from build123d import *

# Parameters (mm, degrees)
BOSS_EXTRUDE1_DEPTH = 3
BOSS_EXTRUDE2_DEPTH = 3
BOSS_EXTRUDE3_DEPTH = 3
BOSS_EXTRUDE4_DEPTH = 3


with BuildPart() as part:
    # Sketch1 → Boss-Extrude1 (new body)
    with BuildSketch(Plane.XY):
        Polygon((0, 0), (5, 1), (1.8, 5.5), (1.8, 1.5), (0, 1.5), align=None)
    extrude(amount=BOSS_EXTRUDE1_DEPTH)

    # Sketch2 → Boss-Extrude2 (add)
    with BuildSketch(Plane(origin=(0, 0, 0), x_dir=(-1, 0, 0), z_dir=(0, 0, -1))):
        Polygon((-5, 1), (-3.2, 3.53125), (-3.2, 1.5), (0, 1.5), (0, 0), align=None)
    extrude(amount=BOSS_EXTRUDE2_DEPTH)

    # Sketch3 → Boss-Extrude3 (add)
    with BuildSketch(Plane(origin=(0, 0, -3), x_dir=(-1, 0, 0), z_dir=(0, 0, -1))):
        Polygon((-3.2, 3.53125), (0, 1.5), (-3.2, 1.5), align=None)
    extrude(amount=-BOSS_EXTRUDE3_DEPTH)

    # Sketch4 → Boss-Extrude4 (add)
    with BuildSketch(Plane.XY):
        Polygon((1.8, 2.642578125), (1.8, 1.5), (0, 1.5), align=None)
    extrude(amount=BOSS_EXTRUDE4_DEPTH)


solid = part.part
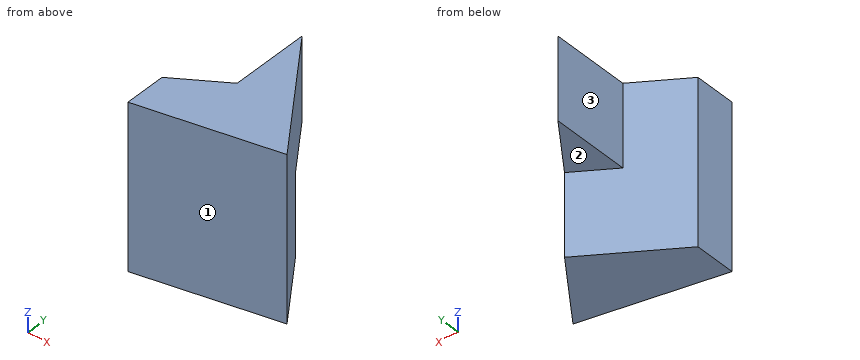
Part model, mm, in its own coordinate system. Face numbers are marked on the shaded views. A direction names the side the tool comes from. Coordinates: 2 decimals unless noted, no trailing zeros. Write each loop counter-clockwise with the first axis right and the second up, starting at its lowest first coordinate (ties: lowest second). Pieces come first, ordered by that corner, then holes. Notation, with made-up numbers: M -9,52 L 37,52 A17 cw 37,85 Z; hole C 0,13 d1. An arc over 180 degrees is marked long. Return JSON: item names as keys, results as strings.
1. Flat gauge pin, fed straight in: pin 1 Ø1.4 at (y, z) = (4.5, 1.5) entering from -X. Where does the tip first touch, or does it go through?
Determined:
{"pin 1": "x = 1.8"}
2. Saw through at C-C, the plane x = 2.55. Write the cut outline in (y, z), then the cut area to 3 significant figures.
Determined:
{"outline": "M 0.51,-3 L 3.12,-3 L 3.12,0 L 4.45,0 L 4.45,3 L 0.51,3 Z", "area": "19.6 mm²"}
3. Saw through at D-D, the plane z = 1.3. Write the cut outline in (x, y).
Determined:
{"outline": "M 0,0 L 5,1 L 1.8,5.5 L 1.8,2.64 L 0,1.5 Z"}
4. Saw through at B-B, the plane y = 4.6. Write the cut outline in (x, z).
Determined:
{"outline": "M 1.8,0 L 2.44,0 L 2.44,3 L 1.8,3 Z"}
5. Saw through at A-A, the plane z = -1.05. Write the cut outline in (x, y), then the cut area to 3 significant figures.
Determined:
{"outline": "M 0,0 L 5,1 L 3.2,3.53 L 0,1.5 Z", "area": "9.63 mm²"}
6. Probe L1, parallel to Y at x = 0.5, z = -1; L2, parallel to Y at x = 2.6, z = 1.05 (3 decimals); L3, parallel to X at y = 3.8, z = 2.7. List the from-to ranges inside material, lowest first.
Determined:
{"L1": "0.1 to 1.82", "L2": "0.52 to 4.375", "L3": "1.8 to 3.01"}
7. 3-axis set-ups, long thin cutter, end or side, ignore diameter. For the marked faces 1, 2 and 3: which of +Z, -Z, +X, -X, +Y, -Y reach the whole face in a straight line?
Determined:
{"face 1": "+Z, -Z, +X, -Y", "face 2": "-Z, -X, +Y", "face 3": "+Z, -Z, -X, +Y"}
